```python
from build123d import *

# Parameters (mm, degrees)
BOSS_EXTRUDE2_DEPTH   = 23
SKETCH1_W             = 20.789980378
SKETCH1_H             = 6
BOSS_EXTRUDE2_2_DEPTH = 23
BOSS_EXTRUDE2_3_DEPTH = 23
BOSS_EXTRUDE2_4_DEPTH = 23
SKETCH1_3_W           = 20.789980378
SKETCH1_3_H           = 36.5
BOSS_EXTRUDE3_DEPTH   = 11
BOSS_EXTRUDE5_DEPTH   = 45
SKETCH2_W             = 9
SKETCH2_H             = 8
CUT_EXTRUDE1_DEPTH    = 106.353028551
SKETCH3_W             = 24.5
SKETCH3_H             = 11
BOSS_EXTRUDE6_DEPTH   = 42
BOSS_EXTRUDE7_DEPTH   = 11
CHAMFER2_SIZE         = 10
SKETCH5_W             = 20.789980378
SKETCH5_H             = 34
CUT_EXTRUDE2_DEPTH    = 104.008391914
SKETCH6_W             = 6
SKETCH6_H             = 12
BOSS_EXTRUDE8_DEPTH   = 22


with BuildPart() as part:
    # Sketch1 → Boss-Extrude2 (new body)
    with BuildSketch(Plane(origin=(0, 0, 0), x_dir=(1, 0, 0), z_dir=(0, 1, 0))):
        Polygon((0.945063883, 6), (0.945063883, 0), (1.890127766, 0), (21.735044261, 0), (21.735044261, 6), align=None)
    extrude(amount=BOSS_EXTRUDE2_DEPTH)



with BuildPart() as body_2:
    # Sketch1 → Boss-Extrude2 2 (new body)
    with BuildSketch(Plane(origin=(0, 0, 0), x_dir=(1, 0, 0), z_dir=(0, 1, 0))):
        with Locations((11.340054072, -15.5)):
            Rectangle(SKETCH1_W, SKETCH1_H)
    extrude(amount=BOSS_EXTRUDE2_2_DEPTH)


with BuildPart() as body_3:
    # Sketch1 → Boss-Extrude2 3 (new body)
    with BuildSketch(Plane(origin=(0, 0, 0), x_dir=(1, 0, 0), z_dir=(0, 1, 0))):
        with Locations((54.13003445, -15.5)):
            Rectangle(SKETCH1_W, SKETCH1_H)
    extrude(amount=BOSS_EXTRUDE2_3_DEPTH)


with BuildPart() as body_4:
    # Sketch1 → Boss-Extrude2 4 (new body)
    with BuildSketch(Plane(origin=(0, 0, 0), x_dir=(1, 0, 0), z_dir=(0, 1, 0))):
        with Locations((54.13003445, 3)):
            Rectangle(SKETCH1_W, SKETCH1_H)
    extrude(amount=BOSS_EXTRUDE2_4_DEPTH)


with BuildPart() as part_1:
    add(part.part)

    add(body_2.part)  # Boss-Extrude3 merges body 2
    # Sketch1<3> → Boss-Extrude3 (add)
    with BuildSketch(Plane(origin=(0, 0, 0), x_dir=(1, 0, 0), z_dir=(0, 1, 0))):
        with Locations((11.340054072, -12.25)):
            Rectangle(SKETCH1_3_W, SKETCH1_3_H)
        with Locations((54.13003445, -12.25)):
            Rectangle(SKETCH1_3_W, SKETCH1_3_H)
    extrude(amount=-BOSS_EXTRUDE3_DEPTH)

    # Sketch1<6> → Boss-Extrude5 (add)
    with BuildSketch(Plane(origin=(0, 0, 0), x_dir=(1, 0, 0), z_dir=(0, 1, 0))):
        Polygon((43.735044261, -18.5), (32.735044261, -18.5), (32.735044261, -60.5), (43.735044261, -60.5), (43.735044261, -30.5), align=None)
        Polygon((32.735044261, -18.5), (21.735044261, -18.5), (21.735044261, -30.5), (21.735044261, -60.5), (32.735044261, -60.5), align=None)
    extrude(amount=-BOSS_EXTRUDE5_DEPTH)

    # Sketch2 → Cut-Extrude1 (cut, through all)
    with BuildSketch(Plane(origin=(74.525024639, 0, 0), x_dir=(0, 0, -1), z_dir=(1, 0, 0))):
        Polygon((-30.5, -11), (-30.5, -3), (-41.183889214, -3), (-57.5, -3), (-57.5, -14.989659462), (-57.5, -41), (-21.5, -41), (-21.5, -11), align=None)
        with Locations((-26, -7)):
            Rectangle(SKETCH2_W, SKETCH2_H)
    extrude(amount=-CUT_EXTRUDE1_DEPTH, mode=Mode.SUBTRACT)


    add(body_3.part)  # Boss-Extrude6 merges body 3

    add(body_4.part)  # Boss-Extrude6 merges body 4
    # Sketch3 → Boss-Extrude6 (add)
    with BuildSketch(Plane.ZY.offset(-43.735044261)):
        with Locations((6.25, -5.5)):
            Rectangle(SKETCH3_W, SKETCH3_H)
    extrude(amount=BOSS_EXTRUDE6_DEPTH)

    # Sketch4 → Boss-Extrude7 (add)
    with BuildSketch(Plane(origin=(0, 0, 0), x_dir=(1, 0, 0), z_dir=(0, 1, 0))):
        Polygon((64.525024639, -18.5), (43.735044261, -18.5), (43.735044261, -12.5), (64.525024639, -12.5), (64.525024639, 0), (43.735044261, 0), (43.735044261, 6), (21.735044261, 6), (21.735044261, 0), (0.945063883, 0), (0.945063883, -12.5), (21.735044261, -12.5), (21.735044261, -18.5), (0.945063883, -18.5), (0.945063883, -30.5), (21.735044261, -30.5), (21.735044261, -60.5), (43.735044261, -60.5), (43.735044261, -30.5), (64.525024639, -30.5), align=None)
    extrude(amount=BOSS_EXTRUDE7_DEPTH)

    # Chamfer2
    chamfer2_edges = [part_1.edges().sort_by_distance(p)[0] for p in [
        (11.340054072, 11, 30.5),
        (32.735044261, 11, 60.5),
        (54.13003445, 11, 30.5),
    ]]
    chamfer(chamfer2_edges, length=CHAMFER2_SIZE)

    # Sketch5 → Cut-Extrude2 (cut, through all)
    with BuildSketch(Plane(origin=(0, 0, -6), x_dir=(-1, 0, 0), z_dir=(0, 0, -1))):
        with Locations((-54.13003445, 6)):
            Rectangle(SKETCH5_W, SKETCH5_H)
    extrude(amount=-CUT_EXTRUDE2_DEPTH, mode=Mode.SUBTRACT)

    # Sketch6 → Boss-Extrude8 (add)
    with BuildSketch(Plane(origin=(21.735044261, 0, 0), x_dir=(0, 0, -1), z_dir=(1, 0, 0))):
        with Locations((-15.5, 17)):
            Rectangle(SKETCH6_W, SKETCH6_H)
        with Locations((3, 17)):
            Rectangle(SKETCH6_W, SKETCH6_H)
    extrude(amount=BOSS_EXTRUDE8_DEPTH)


solid = part_1.part
```
Work out the finished part from the listing and answer in its coordinate system (mm). A direction names the side the tool comes from. Give positions to 0.01 mm unless a question says otherwise; leave off trailing zeros. Order: outer loops, then holes, each group sorted by start corner. A loop starts at its lowest first (then second) coordinate and runs counter-clockwise, first axis right, second up.
1. Each of these flat-tipped pins is pushed along its axis until it touches: P1, Ø11, axis at x = 28.5, y = -26.5, coming from the -Z side; P2, Ø1.5, axis at x = 23, z = 4, coming from the +Y side; P3, Ø6, axis at y = 7.5, z = 30, coming from the -X side. Where does it stop, or does it pass through?
Result sheet:
P1: stops at z = 18.5
P2: stops at y = 11
P3: stops at x = 21.74
2. The mould has two halves that part along Y. Classify faces 1 (the flat face through (33, -41, 40)), 2 (the flat face through (0.945, 2, 8)), 3 (the flat face through (32, 11, 34)): released by +Y, released by -Y, zero draft, split by the parting line, or undercut.
Result sheet:
face 1: undercut
face 2: zero draft
face 3: released by +Y
3. Section A-A, the plane z = 45.5 is taken. Determine the outline of the cut face in (x, y).
Result sheet:
outline: (21.74, -45) - (43.74, -45) - (43.74, -41) - (21.74, -41) - close; (21.74, -3) - (43.74, -3) - (43.74, 11) - (21.74, 11) - close
4. Section D-D, the plane x = 25 is taken. Determine the outline of the cut face in (y, z), and give its area (3 significant figures).
Result sheet:
outline: (-45, 18.5) - (-11, 18.5) - (-11, -6) - (23, -6) - (23, 0) - (11, 0) - (11, 12.5) - (23, 12.5) - (23, 18.5) - (11, 18.5) - (11, 50.5) - (1, 60.5) - (-45, 60.5) - close; hole (-41, 21.5) - (-3, 21.5) - (-3, 57.5) - (-41, 57.5) - close
area: 1,620 mm2
5. Section C-C, the plane x = 15 is taken. Determine the outline of the cut face in (y, z).
Result sheet:
outline: (-11, -6) - (23, -6) - (23, 0) - (11, 0) - (11, 12.5) - (23, 12.5) - (23, 18.5) - (11, 18.5) - (11, 20.5) - (1, 30.5) - (-3, 30.5) - (-3, 21.5) - (-11, 21.5) - close
6. Section B-B, the plane y = -18.5 is taken. Determine the outline of the cut face in (x, z), and give its area (3 significant figures).
Result sheet:
outline: (21.74, 18.5) - (43.74, 18.5) - (43.74, 21.5) - (21.74, 21.5) - close; (21.74, 57.5) - (43.74, 57.5) - (43.74, 60.5) - (21.74, 60.5) - close
area: 132 mm2
7. For faces 4 (the flat face through (11.2, 6.1, 25.4)), 5 (the flat face through (22, 17, 12.5)), 6 (the flat face through (32.6, 6.1, 55.4)), 7 (the flat face through (33, -28, 18.5)), 8 (the flat face through (33, -22, 57.5)), determine the directions among +Z, -Z, +X, -X, +Y, -Y from which every point of the face is accessible in a straight line to the end or side of a thin tool.
Result sheet:
face 4: +Z, -X, +Y
face 5: +X, -X, +Y
face 6: +Z, +X, -X, +Y
face 7: -Z, +X, -X, -Y
face 8: +X, -X
8. Straight lines are drawn through the part: L1, parallel to Y at x = 34.5, z = 43; L2, parallel to Z at x = 40.5, y = -16.5; L3, parallel to Z at x = 40.5, y = 13.5. For each, find the intervals that lie inside material, in ascending order.
Result sheet:
L1: y = -45 to -41, -3 to 11
L2: z = 18.5 to 21.5, 57.5 to 60.5
L3: z = -6 to 0, 12.5 to 18.5
